from build123d import *

# Parameters (mm, degrees)
F0_W     = 28.4
F0_H     = 18.2
F1_DEPTH = 25
F0_W_2   = 22
F0_H_2   = 8
F2_DEPTH = 1.2
F3_R     = 8
F4_DEPTH = 5


with BuildPart() as f1:
    # F0 (on Top) → F1 (new body)
    with BuildSketch(Plane.XY):
        with Locations((0, 5.9)):
            Rectangle(F0_W, F0_H)
        Polygon((11, 2), (13, 2), (13, -2), (-13, -2), (-13, 2), (-11, 2), (-11, 10), (11, 10), align=None, mode=Mode.SUBTRACT)
    extrude(amount=F1_DEPTH)

    # F0 (on Top) → F2 (join)
    with BuildSketch(Plane.XY):
        with Locations((0, 6)):
            Rectangle(F0_W_2, F0_H_2)
        Polygon((13, -2), (13, 2), (11, 2), (-11, 2), (-13, 2), (-13, -2), align=None)
    extrude(amount=F2_DEPTH)

    # F3 (on face) → F4 (cut)
    with BuildSketch(Plane(origin=(0, 15, 0), x_dir=(-1, 0, 0), z_dir=(0, 1, 0))):
        with Locations((0, 10)):
            Circle(F3_R)
    extrude(amount=-F4_DEPTH, mode=Mode.SUBTRACT)


solid = f1.part
The model under review builds one solid part; all positions refer to its coordinate system, in mm. A direction names the side the tool comes from. Round coordinates to 2 decimals unless told otherwise and drop trailing zeros. Loops run counter-clockwise (first coordinate to the right, second up) from the corner with the lowest first, then second, coordinate; pieces in that order, holes last. Notation, with made-up numbers: M 2,6.5 L 45,6.5 A14 ccw 45,20.5 Z; hole C 21,-38 d10. An arc over 180 degrees is marked long. Answer as CSV lines item,"result". Start each with the question number.
Item 1: Consider section D-D (x = -10.25). Write out the cut boundary in (y, z).
Item 2: For faces 4 (the face through (0, -3.2, 12)), 5 (the face through (12, 2, 13)), 6 (the face through (1.73, 12.54, 2.19)), list the 3-axis set-ups (+Z, -Z, +X, -X, +Y, -Y) from which the entire face can be reached by the end or side of a thin tool; tool diameter is ignored.
Item 3: Consider section B-B (z = 10). Write out the cut boundary in (x, y), then the cut area to 3 significant figures.
Item 4: Consider section A-A (x = 0). Write out the cut boundary in (y, z).
Item 5: Mouldability with a two-part tool opening along Y and no side actions: class faces 1 (the face through (-3, 15, 18)), 2 (the face through (13, 0, 13)), 3 (the face through (14.2, 6, 12)) as released by +Y, released by -Y, zero draft, split by the parting line, or undercut.
Item 6: Wall thickness on line 1 (Y direction, x = -7.5, z = 4.5); line 2 (X direction, y = -1, z = 16.25); line 3 (Z direction, x = 0, y = 11.55): over which ranges is each line inside the solid? List them lowest first. Write a range as [from, to].
Item 7: Consider section C-C (y = 12). Write out the cut boundary in (x, z).
Item 8: Insertion check: P1, Ø1.5, axis at x = -1, y = 1.5, coming from the -Z side; P2, Ø6, axis at x = -1.5, y = 5.5, coming from the +Z side. Each pin has a flat end and moves straight along its axis. Give the tip position at first contact, or say it passes through.
Answer:
1,outline,"M -3.2,0 L 15,0 L 15,25 L 10,25 L 10,1.2 L -2,1.2 L -2,25 L -3.2,25 Z"
2,face 4,"+Z, -Z, +X, -X, -Y"
2,face 5,"+Z"
2,face 6,"+Y"
3,outline,"M -14.2,-3.2 L 14.2,-3.2 L 14.2,15 L 8,15 L 8,10 L 11,10 L 11,2 L 13,2 L 13,-2 L -13,-2 L -13,2 L -11,2 L -11,10 L -8,10 L -8,15 L -14.2,15 Z"
3,area,"157 mm^2"
4,outline,"M -3.2,0 L 15,0 L 15,2 L 10,2 L 10,1.2 L -2,1.2 L -2,25 L -3.2,25 Z; M 10,18 L 15,18 L 15,25 L 10,25 Z"
5,face 1,"released by +Y"
5,face 2,"undercut"
5,face 3,"zero draft"
6,line 1,"y = [-3.2, -2], [10, 15]"
6,line 2,"x = [-14.2, -13], [13, 14.2]"
6,line 3,"z = [0, 2], [18, 25]"
7,outline,"M -14.2,0 L 14.2,0 L 14.2,25 L -14.2,25 Z; hole C 0,10 d16"
8,P1,"stops at z = 0"
8,P2,"stops at z = 1.2"
